from build123d import *

# Parameters (mm, degrees)
SKETCH_1_W          = 14
SKETCH_1_H          = 20
EXTRUDE_1_DEPTH     = 3
SKETCH_2_W          = 5
SKETCH_2_H          = 14
CUT_EXTRUDE_1_DEPTH = 3
SKETCH_3_R          = 1
CUT_EXTRUDE_2_DEPTH = 3
SKETCH_4_W          = 2.2
SKETCH_4_H          = 3
CUT_EXTRUDE_3_DEPTH = 3
FILLET_1_R          = 4
FILLET_2_R          = 1
SKETCH_5_R          = 1.25
CUT_EXTRUDE_4_DEPTH = 10


with BuildPart() as part:
    # 스케치1 → 보스-돌출1 (new body)
    with BuildSketch(Plane(origin=(0, 0, 0), x_dir=(0, 0, -1), z_dir=(1, 0, 0))):
        with Locations((7, 10)):
            Rectangle(SKETCH_1_W, SKETCH_1_H)
    extrude(amount=EXTRUDE_1_DEPTH)

    # 스케치2 → 컷-돌출1 (cut)
    with BuildSketch(Plane(origin=(3, 0, 0), x_dir=(0, 0, -1), z_dir=(1, 0, 0))):
        with Locations((7, 10)):
            Rectangle(SKETCH_2_W, SKETCH_2_H)
    extrude(amount=-CUT_EXTRUDE_1_DEPTH, mode=Mode.SUBTRACT)

    # 스케치3 → 컷-돌출2 (cut)
    with BuildSketch(Plane(origin=(3, 0, 0), x_dir=(0, 0, -1), z_dir=(1, 0, 0))):
        with Locations((9.5, 16)):
            Circle(SKETCH_3_R)
        with Locations((4.5, 16)):
            Circle(SKETCH_3_R)
        with Locations((4.5, 4)):
            Circle(SKETCH_3_R)
        with Locations((9.5, 4)):
            Circle(SKETCH_3_R)
    extrude(amount=-CUT_EXTRUDE_2_DEPTH, mode=Mode.SUBTRACT)

    # 스케치4 → 컷-돌출3 (cut)
    with BuildSketch(Plane(origin=(3, 0, 0), x_dir=(0, 0, -1), z_dir=(1, 0, 0))):
        with Locations((7, 1.5)):
            Rectangle(SKETCH_4_W, SKETCH_4_H)
    extrude(amount=-CUT_EXTRUDE_3_DEPTH, mode=Mode.SUBTRACT)

    # 필렛1
    fillet_1_edges = [part.edges().sort_by_distance(p)[0] for p in [
        (1.5, 20, 0),
        (1.5, 20, -14),
        (1.5, 0, -14),
        (1.5, 0, 0),
    ]]
    fillet(fillet_1_edges, radius=FILLET_1_R)

    # 필렛2
    fillet_2_edges = [part.edges().sort_by_distance(p)[0] for p in [
        (1.5, 0, -8.1),
        (1.5, 0, -5.9),
    ]]
    fillet(fillet_2_edges, radius=FILLET_2_R)

    # 스케치5 → 컷-돌출4 (cut)
    with BuildSketch(Plane(origin=(3, 0, 0), x_dir=(0, 0, -1), z_dir=(1, 0, 0))):
        with Locations((7, 17)):
            Circle(SKETCH_5_R)
    extrude(amount=-CUT_EXTRUDE_4_DEPTH, mode=Mode.SUBTRACT)


solid = part.part
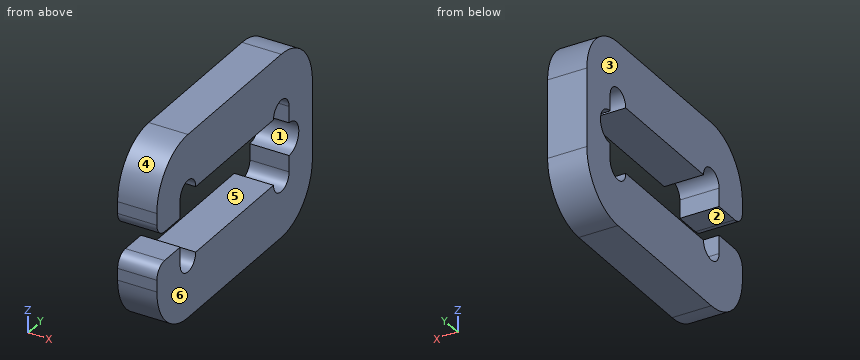
Can you work these out from the model? Positions are in its coordinate system, mm. Face numbers are marked on the shaded views. A direction names the side the tool comes from. Coordinates: 2 decimals unless noted, no trailing zeros. Loops run counter-clockwise (first coordinate to the right, second up) from the corner with the lowest first, then second, coordinate; pieces in that order, holes last. Notation, with made-up numbers: M 57.25,74.25 L 85.25,74.25 A13 cw 85.25,78.25 Z; hole C 8,9 d1. An arc over 180 degrees is marked long. Return JSON: item names as keys, results as strings. Group by question number.
Item 1: I'm going to push a flat-ended pin straight in: pin 1 Ø1 at (x, y) = (1.5, 2) entering from +Z. Where does the tip first touch, or does it pass through?
Item 2: On a 3-axis mill with a long thin cutter (end or side, diameter ignored), from which of +Z, -Z, +X, -X, +Y, -Y can I reach the whole of each face in a straight line? I mean the marked faces 1, 2 and 3. Say none if no direction works.
Item 3: Imagine slicing it at A-A (y = 8.25). Please give me the cut outline in (x, z), and give its area (3 significant figures).
Item 4: Imagine slicing it at B-B (z = -5.5). Please give me the cut outline in (x, y), and give its area (3 significant figures).
Item 5: If I drill on L1, parallel to Z at x = 0.35, y = 11.25; L2, parallel to Z at x = 1.45, y = 16; L3, parallel to Y at x = 1.1, z = -4.75, over which ranges is the centre line in solid material (lowest first)? Write a range as from..to.
Item 6: Imagine slicing it at C-C (x = 1.75). Please give me the cut outline in (y, z).
Item 7: Thinking about a two-plate mould opening in Y: for the marked faces 4, 5 and 6, which applies, released by +Y, released by -Y, zero draft, split by the parting line, or undercut?
Item 8: Imagine slicing it at D-D (z = -10.25). Please give me the cut outline in (x, y).
Verdict:
{
 "1": {"pin 1": "stops at z = -0.29"},
 "2": {"face 1": "+X, -X", "face 2": "+X, -X, -Y", "face 3": "+Z, -Z, -X, +Y, -Y"},
 "3": {"outline": "M 0,-14 L 3,-14 L 3,-9.5 L 0,-9.5 Z; M 0,-4.5 L 3,-4.5 L 3,0 L 0,0 Z", "area": "27.0 mm^2"},
 "4": {"outline": "M 0,0.2 L 3,0.2 L 3,3 L 0,3 Z; M 0,17 L 3,17 L 3,20 L 0,20 Z", "area": "17.4 mm^2"},
 "5": {"L1": "z = -14..-9.5, -4.5..0", "L2": "z = -14..-10.5, -3.5..0", "L3": "y = 0..3, 17..20"},
 "6": {"outline": "M 0,-10 A4 ccw 4,-14 L 16,-14 A4 ccw 20,-10 L 20,-4 A4 ccw 16,0 L 4,0 A4 ccw 0,-4 L 0,-4.9 A1 ccw 1,-5.9 L 3,-5.9 L 3,-4.5 A1 cw 5,-4.5 L 15,-4.5 A1 cw 17,-4.5 L 17,-5.75 A1.25 cw 17,-8.25 L 17,-9.5 A1 cw 15,-9.5 L 5,-9.5 A1 cw 3,-9.5 L 3,-8.1 L 1,-8.1 A1 ccw 0,-9.1 Z"},
 "7": {"face 4": "released by -Y", "face 5": "undercut", "face 6": "zero draft"},
 "8": {"outline": "M 0,0.01 L 3,0.01 L 3,3.34 L 0,3.34 Z; M 0,4.66 L 3,4.66 L 3,15.34 L 0,15.34 Z; M 0,16.66 L 3,16.66 L 3,19.99 L 0,19.99 Z"}
}
